Check sheet for the modelled part. Datum: model origin and axes. Units: mm. Face numbers are marked on the shaded views. A direction names the side the tool comes from. Coordinates: 2 decimals unless noted, no trailing zeros. Loops run counter-clockwise (first coordinate to the right, second up) from the corner with the lowest first, then second, coordinate; pieces in that order, holes last. Notation, with made-up numbers: (46.5, 61) -> (71.5, 61) arc R15 cw to (71.5, 66) -> close; hole circle Ø2 at (60, -16). An arc over 180 degrees is marked (long way). Use one line per item in the form item = value.
from build123d import *

# Parameters (mm, degrees)
BOSS_EXTRUDE1_DEPTH = 2
SKETCH1_3_W         = 17
SKETCH1_3_H         = 7.5
SKETCH1_3_R         = 2.1
BOSS_EXTRUDE2_DEPTH = 11.75
FILLET1_R           = 2
CHAMFER1_SIZE       = 1.5
SKETCH2_W           = 1.5
SKETCH2_H           = 9.75
BOSS_EXTRUDE3_DEPTH = 6
CUT_EXTRUDE1_DEPTH  = 32.102554433
CUT_EXTRUDE2_START  = 11.75
SKETCH1_4_R         = 2.1
CUT_EXTRUDE2_DEPTH  = 5


with BuildPart() as part:
    # Sketch1 → Boss-Extrude1 (new body)
    with BuildSketch(Plane(origin=(0, 0, 0), x_dir=(1, 0, 0), z_dir=(0, 1, 0))):
        with BuildLine():
            ThreePointArc((13.294270592, -2.34784357), (13.448469299, -1.178419919), (13.5, 0))
            Line((13.5, 0), (8.5, 0))
            Line((8.5, 0), (8.5, -7.5))
            Line((8.5, -7.5), (-8.5, -7.5))
            Line((-8.5, -7.5), (-8.5, 0))
            Line((-8.5, 0), (-13.5, 0))
            ThreePointArc((-13.5, 0), (-13.448469299, -1.178419919), (-13.294270592, -2.34784357))
            ThreePointArc((-13.294270592, -2.34784357), (-11.842798665, -2.663810422), (-11.193796958, -4))
            ThreePointArc((-11.193796958, -4), (-11.494084595, -4.964782515), (-12.288862018, -5.588727075))
            ThreePointArc((-12.288862018, -5.588727075), (-8.007808689, -10.86853256), (-1.696626969, -13.392962963))
            ThreePointArc((-1.696626969, -13.392962963), (0, -11.8), (1.696626969, -13.392962963))
            ThreePointArc((1.696626969, -13.392962963), (8.007808689, -10.86853256), (12.288862018, -5.588727075))
            ThreePointArc((12.288862018, -5.588727075), (11.270133638, -3.496296296), (13.294270592, -2.34784357))
        make_face()
        with BuildLine():
            Line((17.5, 0), (13.5, 0))
            ThreePointArc((13.5, 0), (13.448469299, -1.178419919), (13.294270592, -2.34784357))
            ThreePointArc((13.294270592, -2.34784357), (14.229986536, -2.949001707), (14.593796958, -4))
            ThreePointArc((14.593796958, -4), (13.858579473, -5.399712363), (12.288862018, -5.588727075))
            ThreePointArc((12.288862018, -5.588727075), (8.007808689, -10.86853256), (1.696626969, -13.392962963))
            ThreePointArc((1.696626969, -13.392962963), (1.699156533, -13.446454915), (1.7, -13.5))
            ThreePointArc((1.7, -13.5), (-0.053545085, -15.199156533), (-1.696626969, -13.392962963))
            ThreePointArc((-1.696626969, -13.392962963), (-8.007808689, -10.86853256), (-12.288862018, -5.588727075))
            ThreePointArc((-12.288862018, -5.588727075), (-14.517460279, -4.503703704), (-13.294270592, -2.34784357))
            ThreePointArc((-13.294270592, -2.34784357), (-13.448469299, -1.178419919), (-13.5, 0))
            Line((-13.5, 0), (-17.5, 0))
            ThreePointArc((-17.5, 0), (0, -17.5), (17.5, 0))
        make_face()
    extrude(amount=BOSS_EXTRUDE1_DEPTH)

    # Sketch1<3> → Boss-Extrude2 (add)
    # profile 1 of 3: a face of its own
    with BuildSketch(Plane(origin=(0, 0, 0), x_dir=(1, 0, 0), z_dir=(0, 1, 0))):
        with Locations((0, -3.75)):
            Rectangle(SKETCH1_3_W, SKETCH1_3_H)
        with Locations((-4.85, -4.3)):
            Circle(SKETCH1_3_R, mode=Mode.SUBTRACT)
        with Locations((4.85, -4.3)):
            Circle(SKETCH1_3_R, mode=Mode.SUBTRACT)
    # profile 2 of 3: a face of its own
    with BuildSketch(Plane(origin=(0, 0, 0), x_dir=(1, 0, 0), z_dir=(0, 1, 0))):
        with Locations((-4.85, -4.3)):
            Circle(SKETCH1_3_R)
    # profile 3 of 3: a face of its own
    with BuildSketch(Plane(origin=(0, 0, 0), x_dir=(1, 0, 0), z_dir=(0, 1, 0))):
        with Locations((4.85, -4.3)):
            Circle(SKETCH1_3_R)
    extrude(amount=BOSS_EXTRUDE2_DEPTH)

    # Fillet1
    fillet1_edges = [part.edges().sort_by_distance(p)[0] for p in [
        (-17.5, 1, 0),
        (17.5, 1, 0),
        (8.5, 6.875, 7.5),
        (-8.5, 6.875, 7.5),
    ]]
    fillet(fillet1_edges, radius=FILLET1_R)

    # Chamfer1
    chamfer1_edges = [part.edges().sort_by_distance(p)[0] for p in [
        (0, 11.75, 0),
    ]]
    chamfer(chamfer1_edges, length=CHAMFER1_SIZE)

    # Sketch2 → Boss-Extrude3 (add)
    with BuildSketch(Plane.XY.offset(7.5)):
        with Locations((-4.75, 6.875)):
            Rectangle(SKETCH2_W, SKETCH2_H)
        with Locations((4.75, 6.875)):
            Rectangle(SKETCH2_W, SKETCH2_H)
    extrude(amount=BOSS_EXTRUDE3_DEPTH)

    # Sketch3 → Cut-Extrude1 (cut, through all)
    with BuildSketch(Plane(origin=(5.5, 0, 0), x_dir=(0, 0, -1), z_dir=(1, 0, 0))):
        Polygon((-8, 10.25), (-8, 11.75), (-13.5, 11.75), (-13.5, 2.5), (-12, 2.5), align=None)
    extrude(amount=-CUT_EXTRUDE1_DEPTH, mode=Mode.SUBTRACT)

    # Sketch1<4> → Cut-Extrude2 (cut)
    with BuildSketch(Plane(origin=(0, 0, 0), x_dir=(1, 0, 0), z_dir=(0, 1, 0)).offset(CUT_EXTRUDE2_START)):
        with Locations(Location((-4.85, -4.3, 0), (0, 0, 270))):
            Circle(SKETCH1_4_R)
        with Locations(Location((4.85, -4.3, 0), (0, 0, 270))):
            Circle(SKETCH1_4_R)
    extrude(amount=-CUT_EXTRUDE2_DEPTH, mode=Mode.SUBTRACT)


solid = part.part
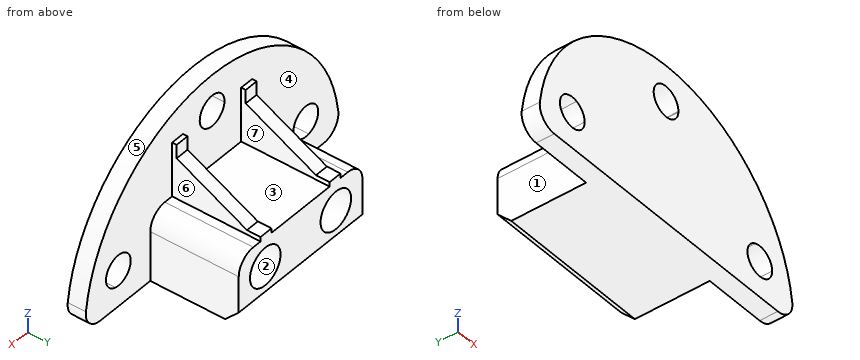
(1) Scan lines: line 1 along X through (y, z) = (10.4, 4.3); line 2 along X through (y, z) = (8.5, 7.75); line 3 along Y through (x, z) = (0, 9.5). Record each from-to range of solid material in increasing order.
Established:
line_1 = -8.5 to -6.95, -2.75 to 2.75, 6.95 to 8.5
line_2 = -5.5 to -4, 4 to 5.5
line_3 = 0 to 2
(2) Section check A-A, the plane y = 1. Record the boundary of the cut face in (x, z), plus the area to 3 significant figures.
Established:
outline = (-17.35, 2.26) arc R2 ccw to (-15.37, 0) -> (15.37, 0) arc R2 ccw to (17.35, 2.26) arc R17.5 ccw to start; hole circle Ø3.4 at (-12.89, 4); hole circle Ø3.4 at (0, 13.5); hole circle Ø3.4 at (12.89, 4)
area = 452 mm²
(3) Go/stop test with flat-tipped pins: P1, Ø3, axis at y = 8, z = 9.5, coming from the -X side; P2, Ø1.6, axis at x = -4.5, z = 13, coming from the +Y side; P3, Ø4, axis at x = -4.85, z = 4.3, coming from the +Y side; P4, Ø6, axis at x = -13, y = 10, coming from the +Z side. Record where each tip stops, or that it passes through.
Established:
P1 = -5.5
P2 = 2.5
P3 = 6.75
P4 = through
(4) Section check C-C, the plane y = 11. Record the boundary of the cut face in (x, z), plus the area to 3 significant figures.
Established:
outline = (-8.5, 0.75) -> (8.5, 0.75) -> (8.5, 5.5) arc R2 ccw to (6.5, 7.5) -> (5.5, 7.5) -> (5.5, 8) -> (4, 8) -> (4, 7.5) -> (-4, 7.5) -> (-4, 8) -> (-5.5, 8) -> (-5.5, 7.5) -> (-6.5, 7.5) arc R2 ccw to (-8.5, 5.5) -> close; hole circle Ø4.2 at (-4.85, 4.3); hole circle Ø4.2 at (4.85, 4.3)
area = 86.8 mm²
(5) Section check B-B, the plane x = 0. Record the boundary of the cut face in (y, z).
Established:
outline = (0, 0) -> (10.25, 0) -> (11.75, 1.5) -> (11.75, 7.5) -> (2, 7.5) -> (2, 11.8) -> (0, 11.8) -> close; (0, 15.2) -> (2, 15.2) -> (2, 17.5) -> (0, 17.5) -> close
(6) Tool access check on the marked faces 1, 2 and 3. Record the directions out of +Z, -Z, +X, -X, +Y, -Y that give a thin tool (end or side, any length) a straight path to the whole face; none if there is none.
Established:
face_1 = +Z, -Z, -X, +Y
face_2 = +Y
face_3 = +Z, +Y
(7) Mould release check, pull along X, two halves, no side actions. Record for the marked faces 4, 5, 6 and 7: +X half, -X half, draft (parallel to the pull), parting line (faces both ways), or undercut.
Established:
face_4 = undercut
face_5 = parting line
face_6 = +X half
face_7 = undercut
(8) Section check D-D, the plane z = 10.5. Record the boundary of the cut face in (x, y), plus the area to 3 significant figures.
Established:
outline = (-14, 0) -> (14, 0) -> (14, 2) -> (5.5, 2) -> (5.5, 5.41) -> (4, 5.41) -> (4, 2) -> (-4, 2) -> (-4, 5.41) -> (-5.5, 5.41) -> (-5.5, 2) -> (-14, 2) -> close
area = 66.2 mm²
